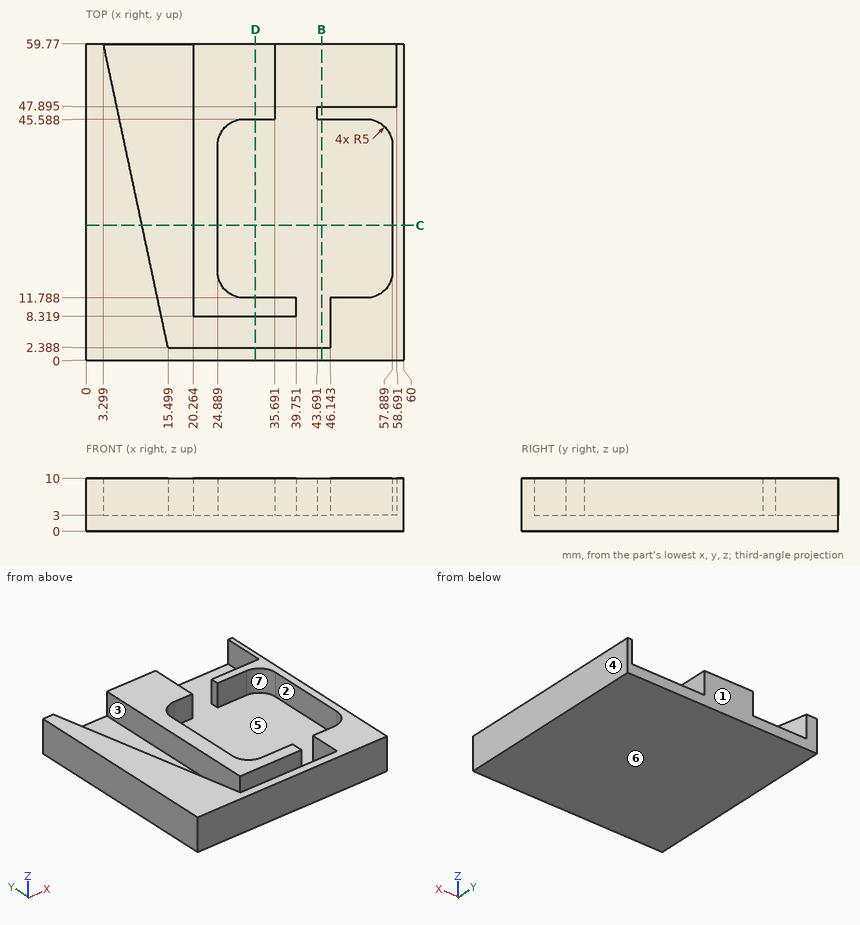
Answer from the drawing. Dimensions are ordinates in mm from the lowest x, y and z of the part. A direction names the side the tool comes from. Give positions to 0.01 mm unless a question says otherwise; leave off trailing zeros. Order: outer loops, then holes, each group sorted by start corner. A loop starts at its lowest first (then second) coordinate and runs counter-clockwise, first axis right, second up.
(1) Given pin 1 (6 mm diameter, centred on x = 38, z = 9, fed in from +Y); pin 2 (5.5 mm diameter, centred on x = 54.5, z = 6, fed in from +Y) (1 decimal); pin 3 (8 mm diameter, centred on x = 32, y = 31, fed in from +Z), each flat-ended and moving along its own axis, determine where each tip first touches the part or whether it passes through.
(2) Find section D-D (x = 32). Give the vertices of the cut face in (y, z).
(3) Straight lines are drawn through the part: L1, parallel to Y at x = 50, z = 3.5 (1 decimal); L2, parallel to Y at x = 22, z = 4.25; L3, parallel to X at y = 30, z = 4.25 (1 decimal). For each, find the intervals that lie inside material, in ascending order.
(4) For a pull along X with two mould halves and no side action, classify the marked faces 4, 5, 6 and 7 as released by +X, released by -X, zero draft, split by the parting line, or undercut.
(5) For the marked faces 1, 2 and 3, determine the directions among +Z, -Z, +X, -X, +Y, -Y from which every point of the face is accessible in a straight line to the end or side of a thin tool.
(6) Find section C-C (y = 25.5). Give the vertices of the cut face in (x, z) (1 decimal).
(7) Find section B-B (x = 44.5). Give the vertices of the cut face in (y, z) (1 decimal).
Result sheet:
1. pin 1: stops at y = 59.77
1. pin 2: stops at y = 47.9
1. pin 3: stops at z = 3
2. outline: (0, 0) - (59.77, 0) - (59.77, 10) - (45.59, 10) - (45.59, 3) - (11.79, 3) - (11.79, 10) - (8.32, 10) - (8.32, 3) - (2.39, 3) - (2.39, 10) - (0, 10) - close
3. L1: y = 0 to 11.8, 45.6 to 47.9
3. L2: y = 0 to 2.39, 8.32 to 59.77
3. L3: x = 0 to 9.6, 20.3 to 24.9, 57.9 to 60
4. face 4: released by +X
4. face 5: undercut
4. face 6: zero draft
4. face 7: undercut
5. face 1: +Z, -Z, +X, -X, +Y
5. face 2: +Z
5. face 3: +Z, +Y
6. outline: (0, 0) - (60, 0) - (60, 10) - (57.9, 10) - (57.9, 3) - (24.9, 3) - (24.9, 10) - (20.3, 10) - (20.3, 3) - (10.6, 3) - (10.6, 10) - (0, 10) - close
7. outline: (0, 0) - (59.8, 0) - (59.8, 3) - (47.9, 3) - (47.9, 10) - (45.6, 10) - (45.6, 3) - (2.4, 3) - (2.4, 10) - (0, 10) - close
